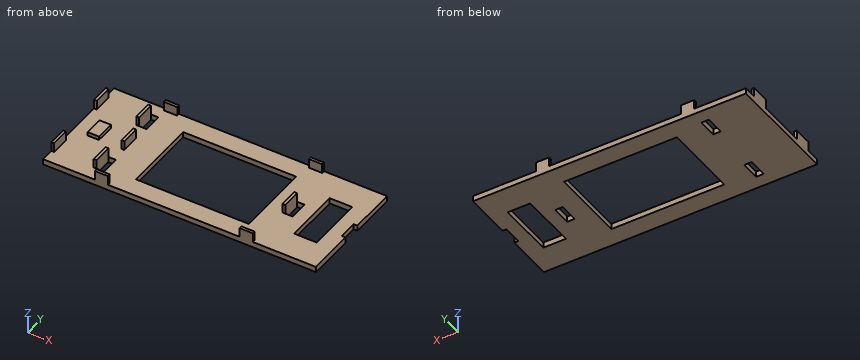
from build123d import *

# Parameters (mm, degrees)
F0_W     = 4
F0_H     = 10
F0_W_2   = 60
F0_H_2   = 40
F0_W_3   = 12
F0_H_3   = 30
F1_DEPTH = 3
F2_W     = 1.5
F2_H     = 10
F2_W_2   = 7
F2_H_2   = 1.5
F3_DEPTH = 5
F4_W     = 6
F4_H     = 10
F5_DEPTH = 2


with BuildPart() as f1:
    # F0 (on Top) → F1 (new body)
    with BuildSketch(Plane.XY):
        Polygon((54.352519, 30), (-90.647481, 30), (-90.647481, -30), (54.352519, -30), (54.352519, -5), (52.352519, -5), (52.352519, 5), (54.352519, 5), align=None)
        with Locations((-64.647481, -18)):
            Rectangle(F0_W, F0_H, mode=Mode.SUBTRACT)
        with Locations((-64.647481, 18)):
            Rectangle(F0_W, F0_H, mode=Mode.SUBTRACT)
        with Locations((-17.647481, 0)):
            Rectangle(F0_W_2, F0_H_2, mode=Mode.SUBTRACT)
        with Locations((24.352519, 0)):
            Rectangle(F0_W, F0_H, mode=Mode.SUBTRACT)
        with Locations((39.352519, 0)):
            Rectangle(F0_W_3, F0_H_3, mode=Mode.SUBTRACT)
    extrude(amount=F1_DEPTH)

    # F2 (on face) → F3 (join)
    with BuildSketch(Plane.XY.offset(3)):
        with Locations((-67.397481, -18)):
            Rectangle(F2_W, F2_H)
        with Locations((-89.897481, -18)):
            Rectangle(F2_W, F2_H)
        with Locations((-67.397481, 18)):
            Rectangle(F2_W, F2_H)
        with Locations((-89.897481, 18)):
            Rectangle(F2_W, F2_H)
        with Locations((-59.647481, -29.25)):
            Rectangle(F2_W_2, F2_H_2)
        with Locations((17.352519, -29.25)):
            Rectangle(F2_W_2, F2_H_2)
        with Locations((-59.647481, 29.25)):
            Rectangle(F2_W_2, F2_H_2)
        with Locations((17.352519, 29.25)):
            Rectangle(F2_W_2, F2_H_2)
        with Locations((21.602519, 0)):
            Rectangle(F2_W, F2_H)
        with Locations((-63.897481, 0)):
            Rectangle(F2_W, F2_H)
    extrude(amount=F3_DEPTH)

    # F4 (on face) → F5 (join)
    with BuildSketch(Plane.XY.offset(3)):
        with Locations((-79.647481, 0)):
            Rectangle(F4_W, F4_H)
    extrude(amount=F5_DEPTH)


solid = f1.part
The model under review builds one solid part; all positions refer to its coordinate system, in mm. Round coordinates to 2 decimals unless told otherwise and drop trailing zeros. Order: outer loops, then holes, each group sorted by start corner. A loop starts at its lowest first (then second) coordinate and runs counter-clockwise, first axis right, second up. Notation, with made-up numbers: (23, 2) -> (52, 2) arc R23 cw to (52, 11) -> close; hole circle Ø3 at (10.25, -34.75). An arc over 180 degrees is marked (long way). Write item = value, one per line. Start each with the question number.
Item 1: Consider section C-C on y = 21.5. Write out the cut boundary in (x, z).
Item 2: Clearance check with flat-ended pins moving along their axes: pin 1 Ø1.5 at (x, z) = (-9.5, 5.5) entering from -Y; pin 2 Ø0.8 at (y, z) = (-29.5, 5.5) entering from +X; pin 3 Ø0.8 at (x, z) = (-90, 5.5) entering from +Y; pin 4 Ø4 at (y, z) = (-17, 5.5) entering from +X. State where each tip first meets the part, or that it passes through.
Item 3: For line 1 along X through (y, z) = (-7.5, 2.5); line 2 along X through (y, z) = (0, 4.75); line 3 along X through (y, z) = (-2, 2.75), list the stretches that pass through material, from the lowest coordinate up.
Item 4: Consider section A-A on y = -2. Write out the cut boundary in (x, z), plus the area to 3 significant figures.
Item 5: Consider section B-B on x = 44. Write out the cut boundary in (y, z), plus the area to 3 significant figures.
Item 6: Consider section D-D on z = 1.25. Write out the cut boundary in (x, y), plus the area to 3 significant figures.
Conclusion:
q1.outline = (-90.65, 0) -> (-66.65, 0) -> (-66.65, 8) -> (-68.15, 8) -> (-68.15, 3) -> (-89.15, 3) -> (-89.15, 8) -> (-90.65, 8) -> close; (-62.65, 0) -> (54.35, 0) -> (54.35, 3) -> (-62.65, 3) -> close
q2.pin_1 = through
q2.pin_2 = 20.85
q2.pin_3 = 23
q2.pin_4 = -66.65
q3.line_1 = -90.65 to -47.65, 12.35 to 33.35, 45.35 to 54.35
q3.line_2 = -82.65 to -76.65, -64.65 to -63.15, 20.85 to 22.35
q3.line_3 = -90.65 to -47.65, 12.35 to 22.35, 26.35 to 33.35, 45.35 to 52.35
q4.outline = (-90.65, 0) -> (-47.65, 0) -> (-47.65, 3) -> (-63.15, 3) -> (-63.15, 8) -> (-64.65, 8) -> (-64.65, 3) -> (-76.65, 3) -> (-76.65, 5) -> (-82.65, 5) -> (-82.65, 3) -> (-90.65, 3) -> close; (12.35, 0) -> (22.35, 0) -> (22.35, 8) -> (20.85, 8) -> (20.85, 3) -> (12.35, 3) -> close; (26.35, 0) -> (33.35, 0) -> (33.35, 3) -> (26.35, 3) -> close; (45.35, 0) -> (52.35, 0) -> (52.35, 3) -> (45.35, 3) -> close
q4.area = 228 mm2
q5.outline = (-30, 0) -> (-15, 0) -> (-15, 3) -> (-30, 3) -> close; (15, 0) -> (30, 0) -> (30, 3) -> (15, 3) -> close
q5.area = 90.0 mm2
q6.outline = (-90.65, -30) -> (54.35, -30) -> (54.35, -5) -> (52.35, -5) -> (52.35, 5) -> (54.35, 5) -> (54.35, 30) -> (-90.65, 30) -> close; hole (-66.65, -23) -> (-62.65, -23) -> (-62.65, -13) -> (-66.65, -13) -> close; hole (-66.65, 13) -> (-62.65, 13) -> (-62.65, 23) -> (-66.65, 23) -> close; hole (-47.65, -20) -> (12.35, -20) -> (12.35, 20) -> (-47.65, 20) -> close; hole (22.35, -5) -> (26.35, -5) -> (26.35, 5) -> (22.35, 5) -> close; hole (33.35, -15) -> (45.35, -15) -> (45.35, 15) -> (33.35, 15) -> close
q6.area = 5,800 mm2
